For this review, use the dimensioned drawing (mm, ordinates from the lowest corner) and the shaded views. A direction names the side the tool comes from. Coordinates: 2 decimals unless noted, no trailing zeros. Loops run counter-clockwise (first coordinate to the right, second up) from the corner with the lowest first, then second, coordinate; pieces in that order, holes last. Notation, with made-up numbers: M 26.25,67.5 L 63.25,67.5 A18 ccw 63.25,71.5 Z; hole C -0.5,56 d8. An arc over 180 degrees is marked long. One line per item, written item: value.
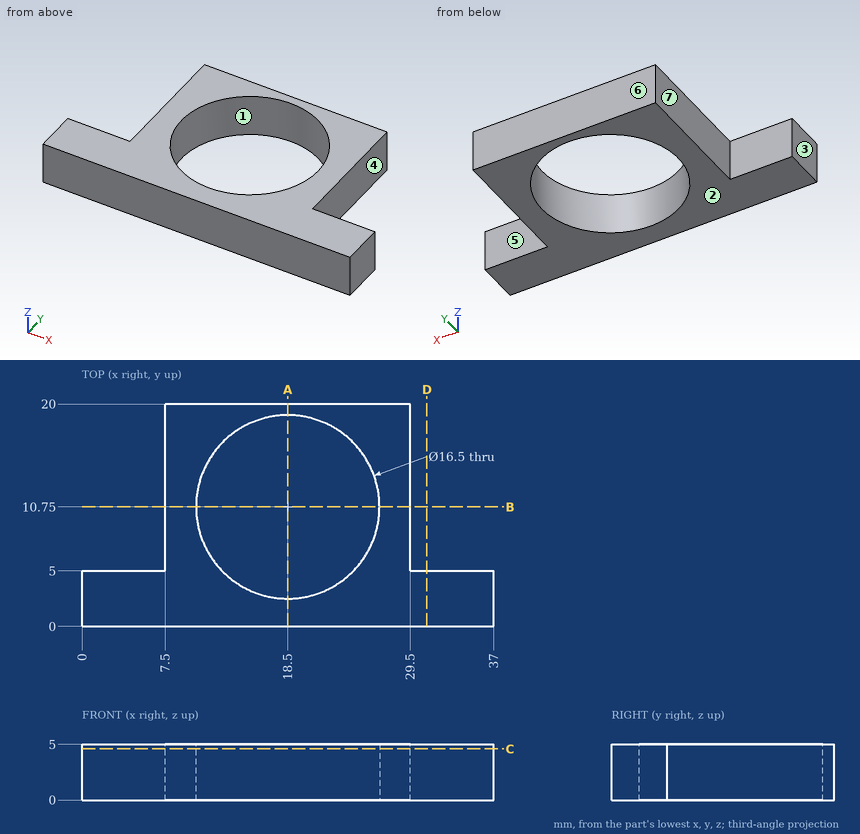
(1) We need section A-A on x = 18.5. State the section outline as (y, z) points, then the cut area to 3 significant figures.
Reply:
outline: M 0,0 L 2.5,0 L 2.5,5 L 0,5 Z; M 19,0 L 20,0 L 20,5 L 19,5 Z
area: 17.5 mm2
(2) We need section B-B on y = 10.75. State the section outline as (x, z) points, then the cut area to 3 significant figures.
Reply:
outline: M 7.5,0 L 10.25,0 L 10.25,5 L 7.5,5 Z; M 26.75,0 L 29.5,0 L 29.5,5 L 26.75,5 Z
area: 27.5 mm2
(3) Insertion check: pin 1 (10 mm diameter, centred on x = 3.5, y = 12.5, fed in from -Z); pin 2 (2.5 mm diameter, centred on y = 13, z = 2, fed in from +X); pin 3 (1.5 mm diameter, centred on y = 11.5, z = 3, fed in from -X). Each pin has a flat end and moves straight along its axis. Give the tip position at first contact, or say it passes through.
Reply:
pin 1: stops at z = 0
pin 2: stops at x = 29.5
pin 3: stops at x = 7.5
(4) We need section D-D on x = 31. State the section outline as (y, z) points, then the cut area to 3 significant figures.
Reply:
outline: M 0,0 L 5,0 L 5,5 L 0,5 Z
area: 25.0 mm2
(5) We need section C-C on z = 4.6. State the section outline as (x, y) points.
Reply:
outline: M 0,0 L 37,0 L 37,5 L 29.5,5 L 29.5,20 L 7.5,20 L 7.5,5 L 0,5 Z; hole C 18.5,10.75 d16.5
(6) To check wall thickness, follow line 1 along Y through (x, z) = (18.5, 3.65); line 2 along Y through (x, z) = (30, 4.85); line 3 along Y through (x, z) = (14, 1.05). State the ranges of each line that lie inside material, in increasing order. Write a range as [from, to].
Reply:
line 1: y = [0, 2.5], [19, 20]
line 2: y = [0, 5]
line 3: y = [0, 3.84], [17.66, 20]
(7) Tool access review of the marked faces 5, 6 and 7: name each direction out of +Z, -Z, +X, -X, +Y, -Y from which nothing blocks a thin tool from reaching the whole face with its end or side.
Reply:
face 5: +Z, -Z, +X, +Y
face 6: +Z, -Z, +X, -X, +Y
face 7: +Z, -Z, -X, +Y
(8) Mouldability with a two-part tool opening along X and no side actions: class the marked faces 1, 2, 3 and 4 as released by +X, released by -X, zero draft, split by the parting line, or undercut.
Reply:
face 1: undercut
face 2: zero draft
face 3: released by -X
face 4: released by +X
